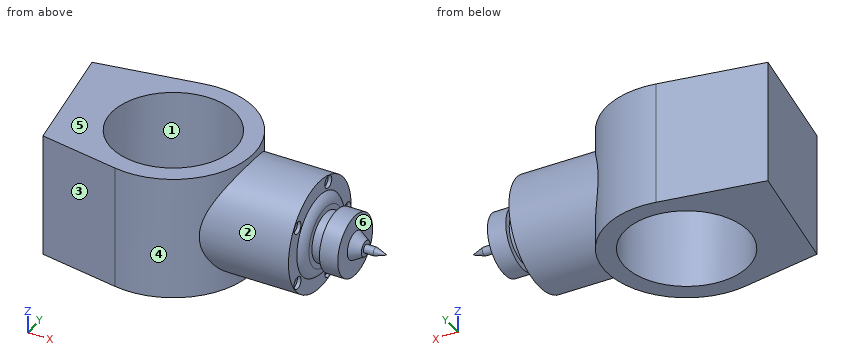
from build123d import *

# Parameters (mm, degrees)
SKETCH1_R                = 50
BOSS_EXTRUDE1_DEPTH      = 50
BOSS_EXTRUDE2_REACH      = 281.962
BOSS_EXTRUDE2_END_RADIUS = 65
SKETCH2_R                = 45
SKETCH4_R                = 5
CUT_EXTRUDE4_DEPTH       = 3
CIRPATTERN2_COUNT        = 5
SKETCH5_R                = 33
BOSS_EXTRUDE3_DEPTH      = 5
FILLET1_R                = 10
SKETCH6_W                = 100
SKETCH6_H                = 80
CUT_EXTRUDE5_DEPTH       = 37
SKETCH7_W                = 37.232866149
SKETCH7_H                = 100
CUT_EXTRUDE6_DEPTH       = 8
SKETCH8_W                = 37
SKETCH8_H                = 100
CUT_EXTRUDE7_DEPTH       = 8
SKETCH9_W                = 16.438055999
SKETCH9_H                = 100
CUT_EXTRUDE8_DEPTH       = 138
CUT_EXTRUDE9_DEPTH       = 138
CUT_EXTRUDE10_DEPTH      = 138


with BuildPart() as part:
    # Sketch1 → Boss-Extrude1 (new, symmetric)
    with BuildSketch(Plane.XY):
        with BuildLine():
            Line((-147.681836523, 40), (-147.681836523, -40))
            Line((-147.681836523, -40), (-11.270034193, -64.015516317))
            ThreePointArc((-11.270034193, -64.015516317), (65, 0), (-11.270034193, 64.015516317))
            Line((-11.270034193, 64.015516317), (-147.681836523, 40))
        make_face()
        with Locations(Location((0, 0, 0), (0, 0, 180))):
            Circle(SKETCH1_R, mode=Mode.SUBTRACT)
    extrude(amount=BOSS_EXTRUDE1_DEPTH, both=True)

    # Boss-Extrude2: up to this cylinder (the profile starts outside it)
    boss_extrude2_end = Plane(origin=(0, 0, 0), z_dir=(0, 0, -1)) * Cylinder(BOSS_EXTRUDE2_END_RADIUS, 694.924, mode=Mode.PRIVATE)
    # Sketch2 → Boss-Extrude2 (add, up to the surface)
    with BuildSketch(Plane(origin=(120, 0, 0), x_dir=(0, 0, -1), z_dir=(1, 0, 0)), mode=Mode.PRIVATE) as boss_extrude2_sk1:
        Circle(SKETCH2_R)
    boss_extrude2_tool1 = extrude(boss_extrude2_sk1.sketch, amount=-BOSS_EXTRUDE2_REACH, mode=Mode.PRIVATE) - boss_extrude2_end
    add(boss_extrude2_tool1.solids().sort_by_distance((120, 0, 0))[0])

    # Sketch3 → Revolve1 (revolve)
    with BuildSketch(Plane.XY, mode=Mode.PRIVATE) as revolve1_sk:
        Polygon((175.096490443, 0), (120, 0), (120, -20), (134, -20), (134, -25), (149, -25), (149, -11.31020279), (157.660254038, -6.31020279), (157.660254038, -3.31020279), (165.660254038, -3.31020279), align=None)
    revolve(revolve1_sk.sketch.rotate(Axis((0, 0, 0), (1, 0, 0)), 270), axis=Axis((0, 0, 0), (1, 0, 0)))

    # Sketch4 → Cut-Extrude4 (cut)
    with BuildSketch(Plane(origin=(120, 0, 0), x_dir=(0, 0, -1), z_dir=(1, 0, 0))):
        with Locations((0, 39.542976343)):
            Circle(SKETCH4_R)
    cut_extrude4 = extrude(amount=-CUT_EXTRUDE4_DEPTH, mode=Mode.SUBTRACT)

    # CirPattern2: Cut-Extrude4 ×5 about axis
    cirpattern2_axis = Axis((0, 0, 0), (1, 0, 0))
    for i in range(1, CIRPATTERN2_COUNT):
        add(cut_extrude4.rotate(cirpattern2_axis, i * 360 / CIRPATTERN2_COUNT), mode=Mode.SUBTRACT)

    # Sketch5 → Boss-Extrude3 (add)
    with BuildSketch(Plane(origin=(120, 0, 0), x_dir=(0, 0, -1), z_dir=(1, 0, 0))):
        Circle(SKETCH5_R)
    extrude(amount=BOSS_EXTRUDE3_DEPTH)

    # Fillet1
    # the kernel refuses this fillet: 10 mm, written as the material it takes off along each edge
    with BuildSketch(Plane(origin=(125, 0, 0), x_dir=(0, 0, -1), z_dir=(0, -1, 0))) as fillet1_piece_1:
        with BuildLine():
            CenterArc((24.339745962, -10), FILLET1_R, 30, 60)
            Line((24.339745962, 0), (24.339745962, 0.2))
            Line((24.339745962, 0.2), (33, 0.2))
            Line((33, 0.2), (33.2, 0))
            ThreePointArc((33.2, 0), (33.2, -2.5), (33.173205081, -4.9))
            Line((33.173205081, -4.9), (33, -5))
        make_face()
    revolve(axis=Axis((125, 0, 0), (1, 0, 0)), mode=Mode.SUBTRACT)

    # Sketch6 → Cut-Extrude5 (cut)
    with BuildSketch(Plane.ZY.offset(147.681836523)):
        Rectangle(SKETCH6_W, SKETCH6_H)
    extrude(amount=-CUT_EXTRUDE5_DEPTH, mode=Mode.SUBTRACT)

    # Sketch7 → Cut-Extrude6 (cut)
    with BuildSketch(Plane(origin=(-11.270034193, 64.015516317, 0), x_dir=(0.9848540971786934, 0.17338514143472855, 0), z_dir=(-0.17338514143472852, 0.9848540971786933, 0))):
        with Locations((-119.893223046, 0)):
            Rectangle(SKETCH7_W, SKETCH7_H)
    extrude(amount=-CUT_EXTRUDE6_DEPTH, mode=Mode.SUBTRACT)

    # Sketch8 → Cut-Extrude7 (cut)
    with BuildSketch(Plane(origin=(0, -40, 0), x_dir=(1, 0, 0), z_dir=(0, 1, 0))):
        with Locations((-129.181836523, 0)):
            Rectangle(SKETCH8_W, SKETCH8_H)
    extrude(amount=-CUT_EXTRUDE7_DEPTH, mode=Mode.SUBTRACT)

    # Sketch9 → Cut-Extrude8 (cut)
    with BuildSketch(Plane(origin=(-11.270034193, 64.015516317, 0), x_dir=(0.9848540971786934, 0.17338514143472855, 0), z_dir=(-0.17338514143472852, 0.9848540971786933, 0))):
        with Locations((-93.057761973, 0)):
            Rectangle(SKETCH9_W, SKETCH9_H)
    extrude(amount=-CUT_EXTRUDE8_DEPTH, mode=Mode.SUBTRACT)


with BuildPart() as cut_extrude8_piece_1:
    # of the separate pieces the step leaves, piece 1, a body of its own (cut_extrude8_pieces)
    add(part.part.solids().sort_by_distance((-11.270034193, 64.015516317, 50))[0])


with BuildPart() as cut_extrude8_piece_2:
    # of the separate pieces the step leaves, piece 2, a body of its own (cut_extrude8_pieces)
    add(part.part.solids().sort_by_distance((-109.625814615, 38.576792986, 50))[0])

    # Sketch10 → Cut-Extrude9 (cut)
    with BuildSketch(Plane.XY.offset(50)):
        Polygon((-110.681836523, -46.51390927), (-110.681836523, 38.390878637), (-107.391706575, 38.390878637), (-90.237190338, -50.805264009), (-110.681836523, -50.805264009), align=None)
    extrude(amount=-CUT_EXTRUDE9_DEPTH, mode=Mode.SUBTRACT)

    # Sketch11 → Cut-Extrude10 (cut)
    with BuildSketch(Plane(origin=(-9.882953062, 56.136683539, 0), x_dir=(0.9848540971786934, 0.17338514143472858, 0), z_dir=(-0.17338514143472855, 0.9848540971786933, 0))):
        Polygon((-96.059625261, -51.911327494), (-97.962360053, 56.770253773), (-112.335310265, 50), (-108.517558636, -51.911327494), align=None)
    extrude(amount=-CUT_EXTRUDE10_DEPTH, mode=Mode.SUBTRACT)


solid = cut_extrude8_piece_1.part
Can you work these out from the model? Positions are in its coordinate system, mm. Face numbers are marked on the shaded views. A direction names the side the tool comes from. Give positions to 0.01 mm unless a question says otherwise; leave off trailing zeros. Order: outer loops, then holes, each group sorted by start corner. A loop starts at its lowest first (then second) coordinate and runs counter-clockwise, first axis right, second up. Notation, with made-up numbers: M 62.5,39.5 L 89.5,39.5 A14 cw 89.5,66.5 Z; hole C -10,28 d7. An arc over 180 degrees is marked long. Use a Markdown table: item, result. Add a question column.
Item 1: Will these pins go through, and if not, where does the flat tip stop? pin 1 (3 mm diameter, centred on y = -32, z = 24.5, fed in from +X); pin 2 (11.5 mm diameter, centred on y = -31.99, z = 23.24, fed in from -X); pin 3 (16 mm diameter, centred on y = 12.22, z = 37.61, fed in from +X); pin 4 (10 mm diameter, centred on y = 0.5, z = 0.5, fed in from +X).
Item 2: Suppose I cut it at A-A (x = 0). List the corners of the cut face in (y, z) for me, then the cut area to 3 significant figures.
Item 3: If I drill on L1, parallel to Y at x = 0, z = 25.5; L2, parallel to X at y = -20, z = -15.5; L3, parallel to Y at x = 37, z = 21, over which ranges is the centre line in solid material (lowest first)? Write a range as [from, to].
Item 4: Suppose I cut it at C-C (x = 61). List the corners of the cut face in (y, z) for me, then the cut area to 3 significant figures.
Item 5: Suppose I cut it at B-B (x = 142.5). List the corners of the cut face in (y, z) for me.
Item 6: We'd pull the mould along X, two halves only. Please class the marked faces 1, 2, 3 and 4: +X half, -X half, draft (parallel to the pull), parting line (faces both ways), or undercut.
Item 7: For the marked faces 5 and 6, which set-ups out of +Z, -Z, +X, -X, +Y, -Y let a thin tool reach every point of the face, with its end or its side?
Answer sheet:
| question | item | result |
|---|---|---|
| 1 | pin 1 | stops at x = 117 |
| 1 | pin 2 | stops at x = -81.52 |
| 1 | pin 3 | stops at x = 121.93 |
| 1 | pin 4 | stops at x = 175.1 |
| 2 | outline | M -65,-50 L -50,-50 L -50,50 L -65,50 Z; M 50,-50 L 65,-50 L 65,50 L 50,50 Z |
| 2 | area | 3,000 mm² |
| 3 | L1 | y = [-65, -50], [50, 65] |
| 3 | L2 | x = [-82.62, -45.83], [45.83, 124.95] |
| 3 | L3 | y = [-53.44, -33.63], [33.63, 53.44] |
| 4 | outline | M -22.45,-50 L 22.45,-50 L 22.45,-39 A45 ccw 22.45,39 L 22.45,50 L -22.45,50 L -22.45,39 A45 ccw -22.45,-39 Z |
| 4 | area | 6,990 mm² |
| 5 | outline | C 0,0 d50 |
| 6 | face 1 | undercut |
| 6 | face 2 | draft |
| 6 | face 3 | -X half |
| 6 | face 4 | parting line |
| 7 | face 5 | +Z, +X, -X, +Y, -Y |
| 7 | face 6 | +X |
